The model under review builds one solid part; all positions refer to its coordinate system, in mm. A direction names the side the tool comes from. Round coordinates to 2 decimals unless told otherwise and drop trailing zeros. Write each loop counter-clockwise with the first axis right and the second up, starting at its lowest first coordinate (ties: lowest second). Pieces come first, ordered by that corner, then holes. Notation, with made-up numbers: (23.5, 21.5) -> (68.5, 21.5) arc R17 ccw to (68.5, 47.5) -> close; hole circle Ø9 at (31.5, 10.5). An arc over 180 degrees is marked (long way). Answer as a JSON object with one key per item and string values. Group by question number.
1) We need section A-A, the plane z = 5.5. Write out the cut boundary in (x, y).
2) We need section C-C, the plane y = 32. Write out the cut boundary in (x, z).
3) We need section B-B, the plane y = 15.5. Write out the cut boundary in (x, z).
4) Machinability: for faces 1 (the flat face through (1, 5, 0)), 2 (the flat face through (-7.5, 2, 1)), 3 (the flat face through (-10, 24.5, 2)), 4 (the flat face through (-12, 28.5, 1)), 5 (the flat face through (-7.5, 17.7, 6.4)), which of the approach directions +Z, -Z, +X, -X, +Y, -Y give a long, thin tool a straight path to every point of the face, cutting with its end or side? Answer none if there is none.
5) Mouldability with a two-part tool opening along Y and no side actions: class faces 6 (the flat face through (0, 45.5, 1)), 7 (the flat face through (-12, 17, 6)), 8 (the flat face through (-7.5, 34, 1)), 9 (the flat face through (-12, 6.5, 1)) as pulls with the +Y half, pulls with the -Y half, needs draft (parallel to the pull), parting line crosses it, or undercut.
6) Insertion check: pin 1 Ø1 at (y, z) = (15.5, 1) entering from -X; pin 2 Ø1 at (x, z) = (-14, 0.5) entering from +Y; pin 3 Ø1 at (x, z) = (-11.5, 5) entering from +Y; pin 4 Ø1 at (x, y) = (-0.5, 21) entering from -Z. Each pin has a flat end and moves straight along its axis. Give the tip position at first contact, or say it passes through.
7) To check wall thickness, follow probe 1 along Y at (x, z) = (-15, 5.5); probe 2 along Z at (x, y) = (5.5, -1); probe 3 along X at (y, z) = (-0.5, 1.25). State the ranges of each line that lie inside material, in increasing order. Write a range as [from, to].
from build123d import *

# Parameters (mm, degrees)
F0_W          = 0.7558596553
F0_H          = 7
F1_DEPTH      = 2
F2_R          = 7
F4_DEPTH      = 2
F5_W          = 4
F5_H          = 2
F6_DEPTH      = 9
F8_DEPTH      = 6
F9_W          = 9
F9_H          = 2
F10_DEPTH     = 14
F11_W         = 4
F11_H         = 2
F12_DEPTH     = 9
F13_W         = 9
F13_H         = 2.5
F14_DEPTH     = 6
F15_T4_DEPTH  = 32.8601958556
F15_T9_DEPTH  = 32.8601958556
F16_T4_DEPTH  = 9
F16_T9_DEPTH  = 9
F16_T11_DEPTH = 19


# Not quite as in the source:
# - a fillet or chamfer that OpenCascade refuses, or shapes differently, is made with other operations: its cross-section is extruded or revolved along the edge and cut away or added
# - a feature names something its author has since deleted; it is built from what else it names


with BuildPart() as f1:
    # F0 (on Top) → F1 (new body)
    with BuildSketch(Plane.XY):
        Polygon((-2.7234070003, 10.5), (-7.5, 10.5), (-7.5, -10.5), (7.5, -10.5), (7.5, 10.5), (1.692557591, 10.5), (0.9366979357, 10.5), (-1.7226199852, 10.5), (-2.5201837998, 10.5), align=None)
        with Locations((1.3146277633, 14)):
            Rectangle(F0_W, F0_H)
        with Locations((1.3146277633, 21)):
            Rectangle(F0_W, F0_H)
        Polygon((-1.7226199852, 24.5), (0.9366979357, 24.5), (1.692557591, 24.5), (7.5, 24.5), (7.5, 45.5), (-7.5, 45.5), (-7.5, 24.5), (-2.7234070003, 24.5), (-2.5201837998, 24.5), align=None)
    extrude(amount=F1_DEPTH)

    # F2
    f2_edges = [f1.edges().sort_by_distance(p)[0] for p in [
        (-7.5, -10.5, 1),
        (7.5, -10.5, 1),
        (7.5, 45.5, 1),
        (-7.5, 45.5, 1),
    ]]
    fillet(f2_edges, radius=F2_R)

    # F3 (on face) → F4 (cut, through all)
    with BuildSketch(Plane.XY.offset(2)):
        with BuildLine():
            ThreePointArc((0, -7), (1.767766953, -6.267766953), (2.5, -4.5))
            ThreePointArc((2.5, -4.5), (1.767766953, -2.732233047), (0, -2))
            Line((0, -2), (0, -4.5))
            Line((0, -4.5), (0, -7))
        make_face()
        with BuildLine():
            ThreePointArc((1, 7.875), (-0.7071067812, 8.5821067812), (0, 6.875))
            ThreePointArc((0, 6.875), (0.7071067812, 7.1678932188), (1, 7.875))
        make_face()
        with BuildLine():
            Line((0, -4.5), (0, -2))
            ThreePointArc((0, -2), (-2.5, -4.5), (0, -7))
            Line((0, -7), (0, -4.5))
        make_face()
        with BuildLine():
            ThreePointArc((2.5, 39.5), (1.767766953, 41.267766953), (0, 42))
            Line((0, 42), (0, 39.5))
            Line((0, 39.5), (0, 37))
            ThreePointArc((0, 37), (1.767766953, 37.732233047), (2.5, 39.5))
        make_face()
        with BuildLine():
            ThreePointArc((1, 27.125), (0.7071067812, 27.8321067812), (0, 28.125))
            ThreePointArc((0, 28.125), (-0.7071067812, 26.4178932188), (1, 27.125))
        make_face()
        with BuildLine():
            Line((0, 39.5), (0, 42))
            ThreePointArc((0, 42), (-2.5, 39.5), (0, 37))
            Line((0, 37), (0, 39.5))
        make_face()
    extrude(amount=-F4_DEPTH, mode=Mode.SUBTRACT)

    # F5 (on face) → F6 (join)
    with BuildSketch(Plane(origin=(-7.5, 0, 0), x_dir=(0, -1, 0), z_dir=(-1, 0, 0))):
        with Locations((-8.5, 1)):
            Rectangle(F5_W, F5_H)
    extrude(amount=F6_DEPTH)

    # F7 (on face) → F8 (join)
    with BuildSketch(Plane.XY.offset(2)):
        Polygon((-8.0660292879, 10.5), (-16.5, 10.5), (-16.5, 8), (-7.5, 8), (-7.5, 10.5), align=None)
    extrude(amount=F8_DEPTH)

    # F9 (on face) → F10 (join)
    with BuildSketch(Plane(origin=(0, 10.5, 0), x_dir=(-1, 0, 0), z_dir=(0, 1, 0))):
        with Locations((12, 7)):
            Rectangle(F9_W, F9_H)
    extrude(amount=F10_DEPTH)

    # F11 (on face) → F12 (join)
    with BuildSketch(Plane(origin=(-7.5, 0, 0), x_dir=(0, -1, 0), z_dir=(-1, 0, 0))):
        with Locations((-26.5, 1)):
            Rectangle(F11_W, F11_H)
    extrude(amount=F12_DEPTH)

    # F13 (on face) → F14 (join)
    with BuildSketch(Plane.XY.offset(2)):
        with Locations((-12, 25.75)):
            Rectangle(F13_W, F13_H)
    extrude(amount=F14_DEPTH)

    # F15: chamfer of 6 on 2 edges, made by hand


with BuildPart() as f15_tool2:
    # F15_s3 → F15_t4 (new body)
    with BuildSketch(Plane.XY.offset(-15.4300979278)):
        Polygon((1.5, 10.5), (7.5, 4.5), (7.5, 10.5), align=None)
    extrude(amount=F15_T4_DEPTH)

    split(bisect_by=Plane.YZ.offset(1.692557591), keep=Keep.TOP)


with BuildPart() as f1_1:
    add(f1.part)

    # F15_t1: cut F15_tool2
    add(f15_tool2.part, mode=Mode.SUBTRACT)


with BuildPart() as f15_tool7:
    # F15_s8 → F15_t9 (new body)
    with BuildSketch(Plane.XY.offset(-15.4300979278)):
        Polygon((7.5, 30.5), (1.5, 24.5), (7.5, 24.5), align=None)
    extrude(amount=F15_T9_DEPTH)

    split(bisect_by=Plane.YZ.offset(1.692557591), keep=Keep.TOP)


with BuildPart() as f1_2:
    add(f1_1.part)

    # F15_t6: cut F15_tool7
    add(f15_tool7.part, mode=Mode.SUBTRACT)

    # F16: fillet of radius 2 on 4 edges, made by hand


with BuildPart() as f16_tool2:
    # F16_s3 → F16_t4 (new body)
    with BuildSketch(Plane.YZ.offset(-16.5)):
        with BuildLine():
            ThreePointArc((8, 4), (7.4142135624, 2.5857864376), (6, 2))
            Line((6, 2), (8, 2))
            Line((8, 2), (8, 4))
        make_face()
    extrude(amount=F16_T4_DEPTH)

    split(bisect_by=Plane.XZ.offset(-6.5), keep=Keep.BOTTOM)


with BuildPart() as f1_3:
    add(f1_2.part)

    # F16_t1: union F16_tool2
    add(f16_tool2.part)


with BuildPart() as f16_tool7:
    # F16_s8 → F16_t9 (new body)
    with BuildSketch(Plane.YZ.offset(-7.5)):
        with BuildLine():
            ThreePointArc((27, 4), (27.5857864376, 2.5857864376), (29, 2))
            Line((29, 2), (27, 2))
            Line((27, 2), (27, 4))
        make_face()
    extrude(amount=-F16_T9_DEPTH)

    split(bisect_by=Plane.XZ.offset(-28.5), keep=Keep.TOP)


with BuildPart() as f1_4:
    add(f1_3.part)

    # F16_t6: union F16_tool7
    add(f16_tool7.part)

    # F16_s12 → F16_t11 (cut)
    with BuildSketch(Plane.YZ.offset(-21.5)):
        with BuildLine():
            ThreePointArc((8, 6), (8.5857864376, 7.4142135624), (10, 8))
            Line((10, 8), (8, 8))
            Line((8, 8), (8, 6))
        make_face()
        with BuildLine():
            ThreePointArc((25, 8), (26.4142135624, 7.4142135624), (27, 6))
            Line((27, 6), (27, 8))
            Line((27, 8), (25, 8))
        make_face()
    extrude(amount=F16_T11_DEPTH, mode=Mode.SUBTRACT)


solid = f1_4.part
Here are the results:
{
 "1": {"outline": "(-16.5, 8) -> (-7.5, 8) -> (-7.5, 10.5) -> (-16.5, 10.5) -> close; (-16.5, 24.5) -> (-7.5, 24.5) -> (-7.5, 27) -> (-16.5, 27) -> close"},
 "2": {"outline": "(-7.5, 0) -> (7.5, 0) -> (7.5, 2) -> (-7.5, 2) -> close"},
 "3": {"outline": "(-16.5, 6) -> (-7.5, 6) -> (-7.5, 8) -> (-16.5, 8) -> close; (0.94, 0) -> (1.69, 0) -> (1.69, 2) -> (0.94, 2) -> close"},
 "4": {"face 1": "-Z, +X, -X, +Y, -Y", "face 2": "+Z, -Z, -X, -Y", "face 3": "-Z, -X", "face 4": "+Z, -Z, -X, +Y", "face 5": "+Z, +X, +Y, -Y"},
 "5": {"face 6": "pulls with the +Y half", "face 7": "undercut", "face 8": "needs draft", "face 9": "pulls with the -Y half"},
 "6": {"pin 1": "stops at x = 0.94", "pin 2": "stops at y = 28.5", "pin 3": "stops at y = 27", "pin 4": "passes through"},
 "7": {"probe 1": "y = [8, 10.5], [24.5, 27]", "probe 2": "z = [0, 2]", "probe 3": "x = [-7.5, 7.5]"}
}
